The figure shows three views and two pictorial views of one solid part (mm, origin at its lowest corner). Answer the questions. A direction names the side the tool comes from. Coordinates: 2 decimals unless noted, no trailing zeros. Order: outer loops, then holes, each group sorted by start corner. A loop starts at its lowest first (then second) coordinate and runs counter-clockwise, first axis right, second up. Notation, with made-up numbers: (-3, 47.5) -> (4, 47.5) arc R19 cw to (4, 80.5) -> close; hole circle Ø7 at (55, -16.75). An arc over 180 degrees is marked (long way). Return JSON: item names as keys, results as strings.
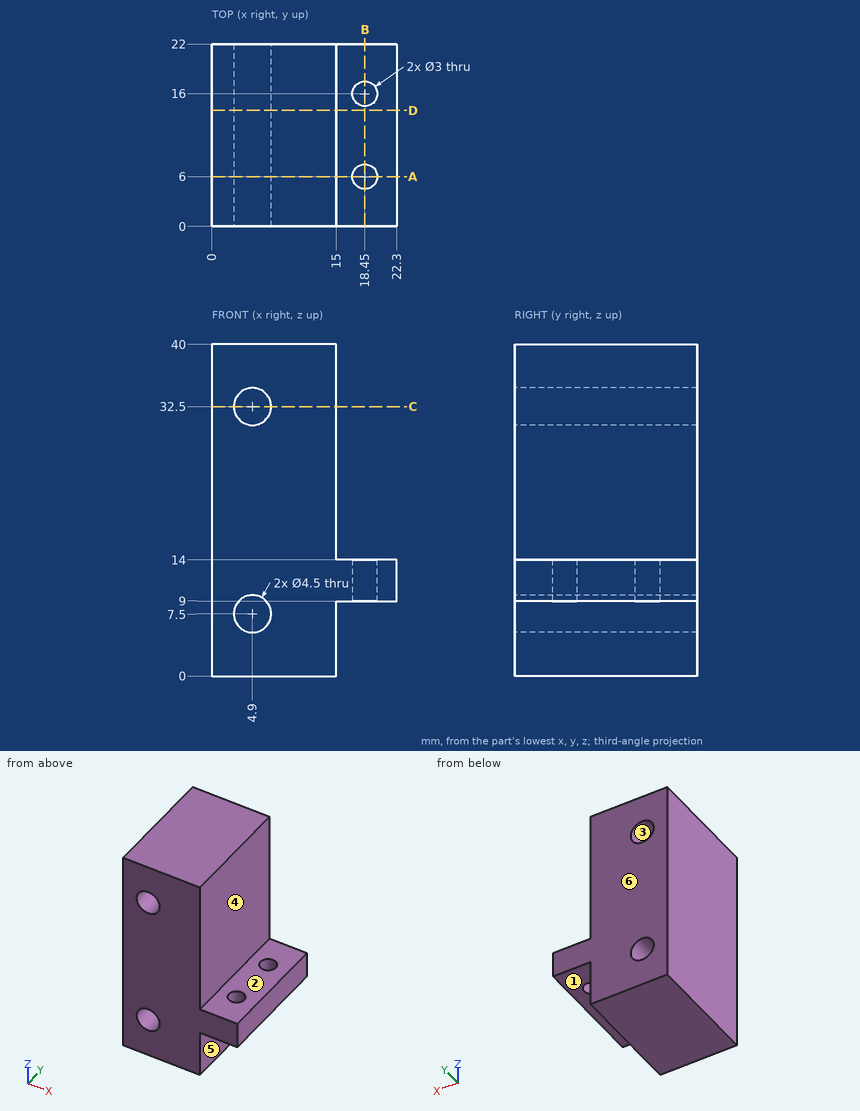
Item 1: Flat-ended cylindrical pins translate along their axes: pin 1 (3.5 mm diameter, centred on x = 18.45, y = 6, fed in from +Z); pin 2 (1.5 mm diameter, centred on x = 5.5, z = 9.5, fed in from -Y); pin 3 (6.5 mm diameter, centred on y = 9.5, z = 26.5, fed in from +X). Find the tip coordinate at first contact, or state that the pin passes through.
Answer list:
{"pin 1": "z = 14", "pin 2": "y = 0", "pin 3": "x = 15"}
Item 2: Find the intervals of material crossed by probe 1 along Y at (x, z) = (18.45, 10.7); probe 2 along Z at (x, y) = (4.9, 15.75); probe 3 along X at (y, z) = (5.5, 4), in increasing order.
Answer list:
{"probe 1": "0 to 4.5, 7.5 to 14.5, 17.5 to 22", "probe 2": "0 to 5.25, 9.75 to 30.25, 34.75 to 40", "probe 3": "0 to 15"}
Item 3: Determine the mould class of the marked faces 1, 2 and 3 for opening direction Z: pulls with the +Z half, pulls with the -Z half, needs draft (parallel to the pull), parting line crosses it, or undercut.
Answer list:
{"face 1": "pulls with the -Z half", "face 2": "pulls with the +Z half", "face 3": "undercut"}
Item 4: Which of the six approach directions +Z, -Z, +X, -X, +Y, -Y give full straight-line access (tool end or side, diameter ignored) to the marked faces 4, 5 and 6?
Answer list:
{"face 4": "+Z, +X, +Y, -Y", "face 5": "-Z, +X, +Y, -Y", "face 6": "+Z, -Z, +X, -X, +Y"}
Item 5: The part is cut by section A-A on y = 6. Determine the outline of the cut face in (x, z), plus the area to 3 significant figures.
Answer list:
{"outline": "(0, 0) -> (15, 0) -> (15, 9) -> (16.95, 9) -> (16.95, 14) -> (15, 14) -> (15, 40) -> (0, 40) -> close; (19.95, 9) -> (22.3, 9) -> (22.3, 14) -> (19.95, 14) -> close; hole circle Ø4.5 at (4.9, 7.5); hole circle Ø4.5 at (4.9, 32.5)", "area": "590 mm2"}
Item 6: The part is cut by section D-D on y = 14. Determine the outline of the cut face in (x, z).
Answer list:
{"outline": "(0, 0) -> (15, 0) -> (15, 9) -> (22.3, 9) -> (22.3, 14) -> (15, 14) -> (15, 40) -> (0, 40) -> close; hole circle Ø4.5 at (4.9, 7.5); hole circle Ø4.5 at (4.9, 32.5)"}
Item 7: The part is cut by section B-B on x = 18.45. Determine the outline of the cut face in (y, z).
Answer list:
{"outline": "(0, 9) -> (4.5, 9) -> (4.5, 14) -> (0, 14) -> close; (7.5, 9) -> (14.5, 9) -> (14.5, 14) -> (7.5, 14) -> close; (17.5, 9) -> (22, 9) -> (22, 14) -> (17.5, 14) -> close"}
Item 8: The part is cut by section C-C on z = 32.5. Determine the outline of the cut face in (x, y).
Answer list:
{"outline": "(0, 0) -> (2.65, 0) -> (2.65, 22) -> (0, 22) -> close; (7.15, 0) -> (15, 0) -> (15, 22) -> (7.15, 22) -> close"}
